from build123d import *


with BuildPart() as part:
    # Skica1 → Rotovat1 (revolve)
    with BuildSketch(Plane(origin=(0, 0, 0), x_dir=(0, 0, -1), z_dir=(1, 0, 0)), mode=Mode.PRIVATE) as rotovat1_sk:
        Polygon((1.288336748, 5.5), (7.288336748, 5.5), (7.288336748, 4), (24.288262464, 4), (24.288262464, 5.5), (30.288262464, 5.5), (30.288262464, 30), (1.288336748, 6.316727332), align=None)
    revolve(rotovat1_sk.sketch.rotate(Axis((0, 0, 59.95975236), (0, 0, -1)), 90), axis=Axis((0, 0, 59.95975236), (0, 0, -1)))


solid = part.part
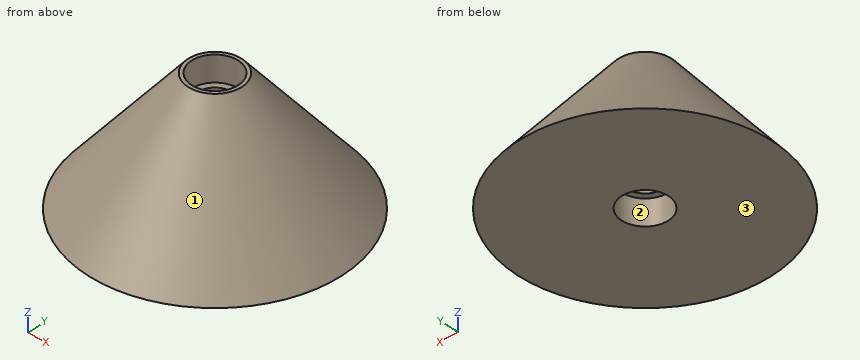
Here's how the part is built. I have some questions about the finished solid (model axes, mm). Face numbers are marked on the shaded views. Give positions to 0.01 mm unless a question says otherwise; leave off trailing zeros. Loops run counter-clockwise (first coordinate to the right, second up) from the corner with the lowest first, then second, coordinate; pieces in that order, holes last. Notation, with made-up numbers: (-12.5, 61.25) -> (10.5, 61.25) arc R19 ccw to (10.5, 97.25) -> close; hole circle Ø8 at (73.5, 15.25). An arc over 180 degrees is marked (long way). One line per item, written item: value.
Q1. Suppose I cut it at A-A on x = 0. Please give me the cut outline in (y, z), then the cut area to 3 significant figures.
Answers follow:
outline: (-30, -30.29) -> (-5.5, -30.29) -> (-5.5, -24.29) -> (-4, -24.29) -> (-4, -7.29) -> (-5.5, -7.29) -> (-5.5, -1.29) -> (-6.32, -1.29) -> close; (4, -24.29) -> (5.5, -24.29) -> (5.5, -30.29) -> (30, -30.29) -> (6.32, -1.29) -> (5.5, -1.29) -> (5.5, -7.29) -> (4, -7.29) -> close
area: 785 mm^2
Q2. Suppose I cut it at D-D on z = -4.75. Please give me the cut outline in (x, y), then the cut area to 3 significant figures.
Answers follow:
outline: circle Ø18.29 at (0, 0); hole circle Ø11 at (0, 0)
area: 168 mm^2
Q3. I'm going to push flat-ended pins straight in: pin 1 Ø12 at (x, z) = (19, -13) entering from -Y; pin 2 Ø3.5 at (x, y) = (-2.5, 0.5) entering from +Z; pin 3 Ø6 at (x, z) = (5.5, -12) entering from -Y; pin 4 Ø6.5 at (x, y) = (0, 0) entering from -Z. Where does each tip first touch, or does it pass through?
Answers follow:
pin 1: y = -12.52
pin 2: z = -7.29
pin 3: y = -16.78
pin 4: through
Q4. We'd pull the mould along X, two halves only. Please class the marked faces 1, 2 and 3: pulls with the +X half, pulls with the -X half, needs draft (parallel to the pull), parting line crosses it, or undercut.
Answers follow:
face 1: parting line crosses it
face 2: undercut
face 3: needs draft
Q5. Suppose I cut it at C-C on z = -9.25. Please give me the cut outline in (x, y), then the cut area to 3 significant figures.
Answers follow:
outline: circle Ø25.64 at (0, 0); hole circle Ø8 at (0, 0)
area: 466 mm^2
Q6. If I drill on line 1 along X through (y, z) = (-4.5, -2.75); line 2 along Y through (x, z) = (0, -19.5); line 3 along Y through (x, z) = (0, -2.75), over which ranges is the centre line in solid material (lowest first)?
Answers follow:
line 1: -6.01 to -3.16, 3.16 to 6.01
line 2: -21.19 to -4, 4 to 21.19
line 3: -7.51 to -5.5, 5.5 to 7.51
